Geometry: see drawing. Coordinates: mm, zero at the bounding-box minimum. A direction names the side the tool comes from. Coordinates: 2 decimals unless noted, no trailing zeros. Loops run counter-clockwise (first coordinate to the right, second up) from the corner with the lowest first, then second, coordinate; pieces in that order, holes last. Notation, with made-up numbers: (-36, -10) -> (11, -10) arc R23 ccw to (11, 27) -> close; hole circle Ø6 at (5, 6). An arc over 180 degrees is marked (long way). One line per question, with ' | ' between items. Start each with the question number.
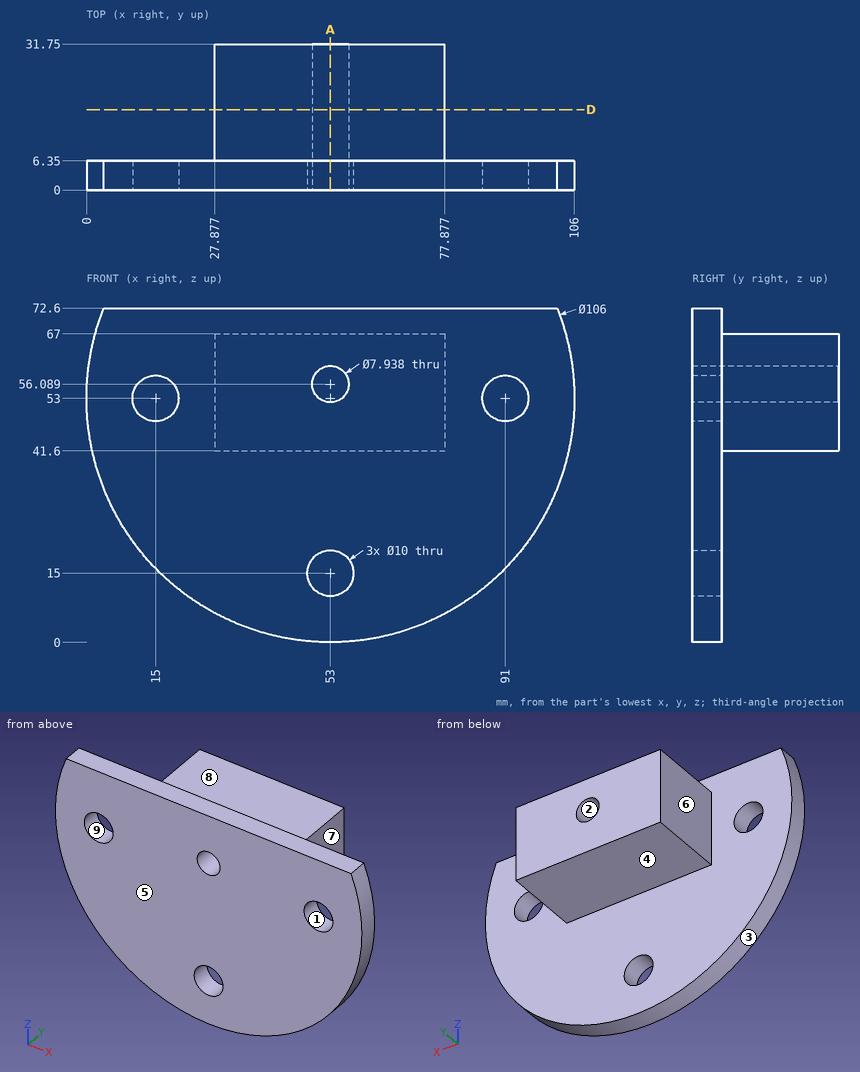
(1) Cut plane A-A, the plane x = 53. Return the cut outline in (y, z).
(2) Access query for the marked faces 5, 6, 7, 8 and 9. Directions: +Z, -Z, +X, -X, +Y, -Y. A direction counts if a zero-diameter tool reaches every point of the face in a straight line with its end or side. Return the directions, or none.
(3) Contact query for flat-ended pins moving along their axis: pin 1 Ø3 at (y, z) = (17.5, 44) entering from -X; pin 2 Ø7 at (x, z) = (53, 56.09) entering from +Y; pin 3 Ø16 at (x, z) = (91, 53) entering from +Y; pin 4 Ø5 at (y, z) = (13, 43.5) entering from +X. Output: stop coordinate, or through.
(4) Draft query along X for the marked faces 1, 2, 3 and 4. Return one class per face: pulls with the +X half, pulls with the -X half, needs draft (parallel to the pull), parting line crosses it, or undercut.
(5) Ray query, L1, parallel to Z at x = 53, y = 3; L2, parallel to X at y = 2, z = 53; L3, parallel to Y at x = 80, z = 61. Return the intervals inside material, ascending.
(6) Cut plane D-D, the plane y = 17.5. Return the cut outline in (x, z).
Here are the results:
1) outline: (0, 0) -> (6.35, 0) -> (6.35, 10) -> (0, 10) -> close; (0, 20) -> (6.35, 20) -> (6.35, 41.6) -> (31.75, 41.6) -> (31.75, 52.12) -> (0, 52.12) -> close; (0, 60.06) -> (31.75, 60.06) -> (31.75, 67) -> (6.35, 67) -> (6.35, 72.6) -> (0, 72.6) -> close
2) face 5: +Z, -Z, +X, -X, -Y | face 6: +Z, -Z, -X, +Y | face 7: +Z, -Z, +X, +Y | face 8: +Z, +X, -X, +Y | face 9: +Y, -Y
3) pin 1: stops at x = 27.88 | pin 2: passes through | pin 3: stops at y = 6.35 | pin 4: stops at x = 77.88
4) face 1: undercut | face 2: undercut | face 3: parting line crosses it | face 4: needs draft
5) L1: z = 0 to 10, 20 to 52.12, 60.06 to 72.6 | L2: x = 0 to 10, 20 to 50.51, 55.49 to 86, 96 to 106 | L3: y = 0 to 6.35
6) outline: (27.88, 41.6) -> (77.88, 41.6) -> (77.88, 67) -> (27.88, 67) -> close; hole circle Ø7.94 at (53, 56.09)
